Check sheet for the modelled part. Datum: model origin and axes. Units: mm. Round coordinates to 2 decimals unless told otherwise and drop trailing zeros. Write each loop counter-clockwise with the first axis right and the second up, starting at its lowest first coordinate (ties: lowest second). Pieces come first, ordered by that corner, then holes.
Item 1: Go/stop test with flat-tipped pins: pin 1 Ø7 at (x, y) = (71, 20) entering from -Z; pin 2 Ø1.8 at (x, z) = (27.5, 3.5) entering from +Y; pin 3 Ø1.6 at (y, z) = (89, 4) entering from -X. Record where each tip stops, or that it passes through.
Item 2: Cross-section at D-D on y = 51. Enter the section's corners in (x, z).
Item 3: Material ranges on line 1 (Y direction, x = 31.5, z = 2.5); line 2 (Y direction, x = 50, z = 4.7); line 3 (Y direction, x = 14, z = 4.55), recorded low to high.
Item 4: Cross-section at A-A on y = 20. Enter the section's corners in (x, z).
Item 5: Cross-section at B-B on x = 6. Enter the section's corners in (y, z).
Item 6: Cross-section at C-C on x = 14. Enter the section's corners in (y, z), plus the area to 3 significant figures.
Autodesk Inventor part; units mm, degrees
ref_plane "YZ Plane" through (0, 0, 0) normal (1, 0, 0) x (0, 1, 0)
ref_plane "XZ Plane" through (0, 0, 0) normal (0, 1, 0) x (-1, 0, 0)
ref_plane "XY Plane" through (0, 0, 0) normal (0, 0, 1) x (1, 0, 0)
sketch "Sketch1" plane through (0, 0, 0) normal (0, 0, 1) x (1, 0, 0)
  line L0 (0, 0) -> (68, 0)
  line L1 (68, 86) -> (0, 86)
  line L2 (0, 86) -> (0, 0)
  line L3 (68, 71) -> (78, 61)
  line L4 (78, 61) -> (78, 19)
  line L5 (78, 19) -> (68, 9)
  line L6 (68, 0) -> (68, 9)
  line L7 (68, 71) -> (68, 86)
  line L8 (37.5, 83) -> (45.5, 83)
  line L9 (45.5, 83) -> (45.5, 77)
  line L10 (45.5, 77) -> (37.5, 77)
  line L11 (37.5, 77) -> (37.5, 83)
  line L12 (10, 77) -> (18, 77)
  line L13 (18, 77) -> (18, 71)
  line L14 (18, 71) -> (10, 71)
  line L15 (10, 71) -> (10, 77)
  line L16 (10, 9) -> (18, 9)
  line L17 (18, 9) -> (18, 3)
  line L18 (18, 3) -> (10, 3)
  line L19 (10, 3) -> (10, 9)
  line L20 (25, 70) -> (34, 70)
  line L21 (35, 69) -> (35, 46)
  line L22 (34, 45) -> (25, 45)
  line L23 (24, 46) -> (24, 69)
  line L24 (25, 35) -> (34, 35)
  line L25 (35, 34) -> (35, 11)
  line L26 (34, 10) -> (25, 10)
  line L27 (24, 11) -> (24, 34)
  arc A0 (25, 70) -> (24, 69) centre (25, 69) ccw
  arc A1 (35, 69) -> (34, 70) centre (34, 69) ccw
  arc A2 (34, 45) -> (35, 46) centre (34, 46) ccw
  arc A3 (24, 46) -> (25, 45) centre (25, 46) ccw
  arc A4 (25, 35) -> (24, 34) centre (25, 34) ccw
  arc A5 (24, 11) -> (25, 10) centre (25, 11) ccw
  arc A6 (34, 10) -> (35, 11) centre (34, 11) ccw
  arc A7 (35, 34) -> (34, 35) centre (34, 34) ccw
  line L28 (29.5, 70) -> (29.5, 10) construction
  circle A8 centre (71, 60) radius 2.75
  circle A9 centre (71, 20) radius 2.75
  line L29 (48.5, 3) -> (56.5, 3)
  line L30 (56.5, 3) -> (56.5, 9)
  line L31 (56.5, 9) -> (48.5, 9)
  line L32 (48.5, 9) -> (48.5, 3)
  circle A10 centre (6, 13) radius 5 construction
  circle A11 centre (6, 13) radius 2.75
  circle A12 centre (6, 67) radius 5 construction
  circle A13 centre (6, 67) radius 2.75
  line L33 (48.5, 77) -> (56.5, 77)
  line L34 (56.5, 77) -> (56.5, 71)
  line L35 (56.5, 71) -> (48.5, 71)
  line L36 (48.5, 71) -> (48.5, 77)
  line L37 (21, 83) -> (29, 83)
  line L38 (29, 83) -> (29, 77)
  line L39 (29, 77) -> (21, 77)
  line L40 (21, 77) -> (21, 83)
  circle A14 centre (71, 60) radius 5 construction
  circle A15 centre (71, 20) radius 5 construction
  circle A16 centre (14, 40) radius 5 construction
  circle A17 centre (46, 40) radius 5 construction
  circle A18 centre (46, 40) radius 2.75
  circle A19 centre (14, 40) radius 2.75
  line L41 (50, 86) -> (50, 0) construction
  line L42 (55, 86) -> (55, 0) construction
  line L43 (52.5, 86) -> (52.5, 0) construction
  point P0 (78, 40)
  dimension "d1" = 45
  dimension "d2" = 10
  dimension "d3" = 6
  dimension "d4" = 6
  dimension "d5" = 8
  dimension "d6" = 8
  dimension "d7" = 3
  dimension "d8" = 6
  dimension "d9" = 3
  dimension "d12" = 1
  dimension "d13" = 11
  dimension "d14" = 25
  dimension "d15" = 25
  dimension "d16" = 1
  dimension "d17" = 1
  dimension "d18" = 38.5
  dimension "d19" = 5.5
  dimension "d20" = 5.5
  dimension "d21" = 7
  dimension "d23" = 6
  dimension "d24" = 8
  dimension "d25" = 11
  dimension "d26" = 11
  dimension "d27" = 10
  dimension "d28" = 5.5
  dimension "d29" = 5.5
  dimension "d30" = 10
  dimension "d32" = 4
  dimension "d33" = 4
  dimension "d34" = 4
  dimension "d35" = 6
  dimension "d36" = 68
  dimension "d37" = 11.5
  dimension "d38" = 3
  dimension "d39" = 8
  dimension "d40" = 3
  dimension "d41" = 10
  dimension "d42" = 10
  dimension "d43" = 4
  dimension "d44" = 10
  dimension "d45" = 5.5
  dimension "d46" = 10
  dimension "d47" = 5.5
  dimension "d49" = 14
  dimension "d50" = 32
  dimension "d51" = 5
  dimension "d52" = 2.5
  dimension "d53" = 15.5
  dimension "d69" = 86
extrude "Extrusion1" add sketch "Sketch1" along normal blind 6
chamfer "Chamfer1" distance 2 angle 45 4 edges at (0, 0, 3) (68, 0, 3) (68, 86, 3) (0, 86, 3)
sketch "Sketch2" plane through (0, 0, 6) normal (0, 0, 1) x (1, 0, 0)
  line L0 (48.5, 9) -> (56.5, 9)
  line L1 (68, 2) -> (68, 9)
  line L2 (48.5, 15) -> (56.5, 15)
  line L3 (56.5, 15) -> (56.5, 9)
  line L4 (56.5, 9) -> (48.5, 9)
  line L5 (48.5, 9) -> (48.5, 15)
  point P0 (0, 0)
  dimension "d59" = 6
  dimension "d60" = 8
  dimension "d63" = 11.5
extrude "Extrusion2" cut sketch "Sketch2" against normal through all
sketch "Sketch3" plane through (0, 0, 6) normal (0, 0, 1) x (1, 0, 0)
  line L0 (29, 83) -> (29, 77)
  line L1 (29, 77) -> (21, 77)
  line L2 (21, 77) -> (21, 83)
  line L3 (21, 83) -> (29, 83)
  point P0 (0, 0)
extrude "Extrusion3" add sketch "Sketch3" against normal blind 6
sketch "Sketch6" plane through (0, 0, 6) normal (0, 0, 1) x (1, 0, 0)
  line L0 (56.5, 77) -> (56.5, 71)
  line L1 (48.5, 71) -> (48.5, 77)
  line L2 (18, 77) -> (18, 71)
  line L3 (10, 71) -> (10, 77)
  line L4 (66, 86) -> (2, 86)
  line L5 (7, 86) -> (21, 86)
  line L6 (21, 86) -> (21, 92)
  line L7 (21, 92) -> (7, 92)
  line L8 (7, 92) -> (7, 86)
  line L9 (45.5, 86) -> (59.5, 86)
  line L10 (59.5, 86) -> (59.5, 92)
  line L11 (59.5, 92) -> (45.5, 92)
  line L12 (45.5, 92) -> (45.5, 86)
  point P0 (0, 0)
  dimension "d80" = 3
  dimension "d81" = 3
  dimension "d82" = 3
  dimension "d83" = 3
  dimension "d84" = 6
extrude "Extrusion6" add sketch "Sketch6" against normal blind 6
sketch "Sketch7" plane through (0, 0, 6) normal (0, 0, 1) x (1, 0, 0)
  line L0 (56.5, 77) -> (56.5, 71)
  line L1 (48.5, 71) -> (48.5, 77)
  line L2 (18, 77) -> (18, 71)
  line L3 (10, 71) -> (10, 77)
  line L4 (45.5, 83) -> (45.5, 77)
  line L5 (37.5, 77) -> (37.5, 83)
  line L6 (37.5, 83) -> (45.5, 83)
  line L7 (10, 89) -> (18, 89)
  line L8 (18, 89) -> (18, 83)
  line L9 (18, 83) -> (10, 83)
  line L10 (10, 83) -> (10, 89)
  line L11 (48.5, 89) -> (56.5, 89)
  line L12 (56.5, 89) -> (56.5, 83)
  line L13 (56.5, 83) -> (48.5, 83)
  line L14 (48.5, 83) -> (48.5, 89)
  point P0 (0, 0)
extrude "Extrusion7" cut sketch "Sketch7" against normal blind 6
chamfer "Chamfer3" distance 2 angle 45 8 edges at (7, 86, 3) (7, 92, 3) (21, 92, 3) (21, 86, 3) (45.5, 86, 3) (45.5, 92, 3) (59.5, 92, 3) (59.5, 86, 3)
properties part number "x_motor_top"
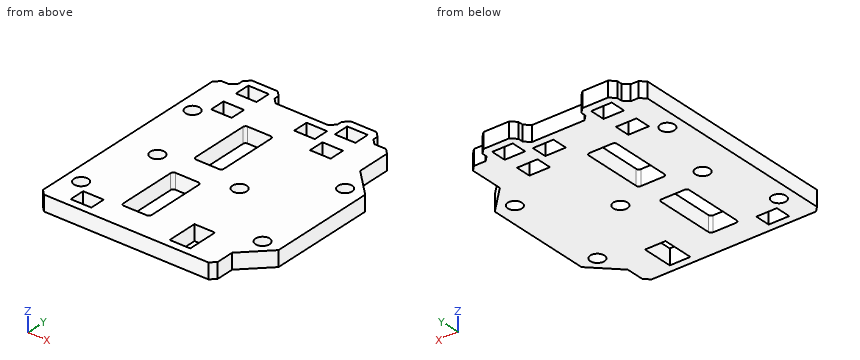
Response values:
1. pin 1: stops at z = 0
1. pin 2: stops at y = 86
1. pin 3: stops at x = 7
2. outline: (0, 0) - (24, 0) - (24, 6) - (0, 6) - close; (35, 0) - (78, 0) - (78, 6) - (35, 6) - close
3. line 1: y = 0 to 10, 35 to 45, 70 to 86
3. line 2: y = 0 to 3, 15 to 71, 77 to 83, 89 to 92
3. line 3: y = 0 to 3, 9 to 37.25, 42.75 to 71, 77 to 83, 89 to 92
4. outline: (0, 0) - (24, 0) - (24, 6) - (0, 6) - close; (35, 0) - (68.25, 0) - (68.25, 6) - (35, 6) - close; (73.75, 0) - (78, 0) - (78, 6) - (73.75, 6) - close
5. outline: (0, 0) - (10.25, 0) - (10.25, 6) - (0, 6) - close; (15.75, 0) - (64.25, 0) - (64.25, 6) - (15.75, 6) - close; (69.75, 0) - (87, 0) - (87, 6) - (69.75, 6) - close
6. outline: (0, 0) - (3, 0) - (3, 6) - (0, 6) - close; (9, 0) - (37.25, 0) - (37.25, 6) - (9, 6) - close; (42.75, 0) - (71, 0) - (71, 6) - (42.75, 6) - close; (77, 0) - (83, 0) - (83, 6) - (77, 6) - close; (89, 0) - (92, 0) - (92, 6) - (89, 6) - close
6. area: 411 mm2
